Here's the drawing with two shaded views (mm, measured from the low corner). I have some questions. A direction names the side the tool comes from. Give positions to 0.01 mm unless a question says otherwise; leave off trailing zeros. Write each loop counter-clockwise with the first axis right and the second up, starting at its lowest first coordinate (ties: lowest second). Pieces come first, ordered by that corner, then holes. Notation, with made-up numbers: M 37.5,64 L 58.5,64 A5 cw 58.5,72 Z; hole C -14.5,48.25 d2. An arc over 180 degrees is marked long. Use one line per item in the form item = value.
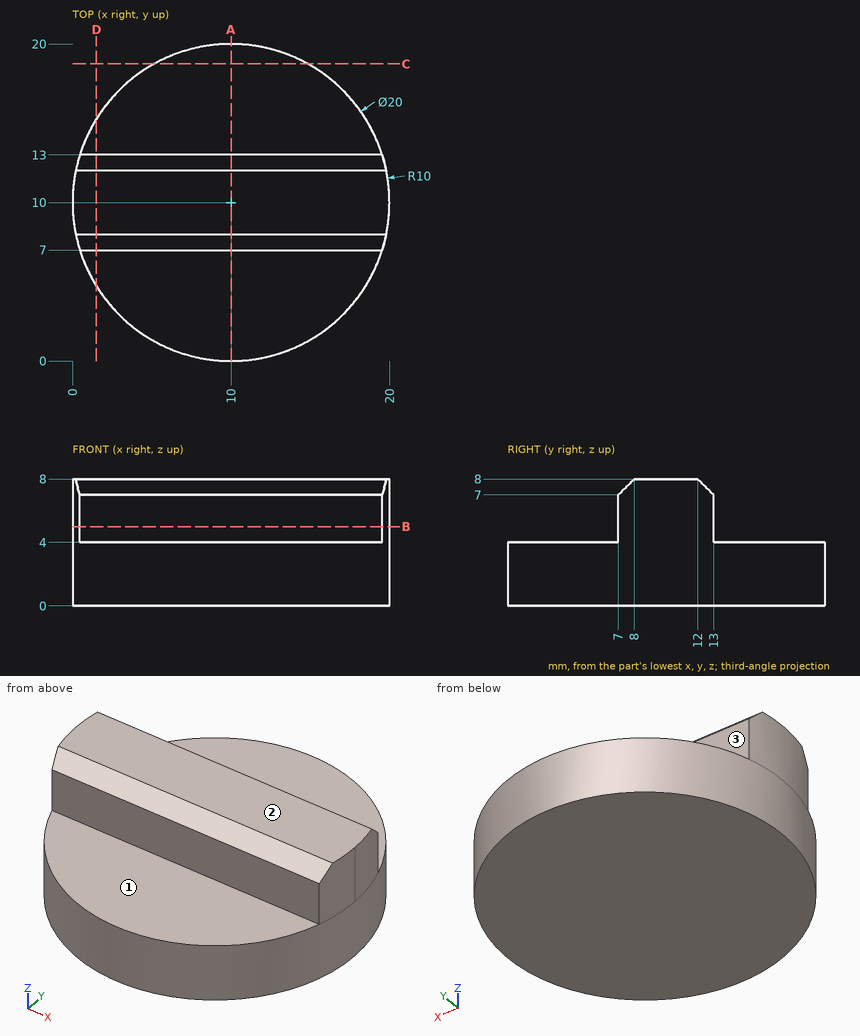
1) For pin 1 Ø2.5 at (x, z) = (10.5, 5) entering from +Y; pin 2 Ø1.5 at (x, z) = (6, 5.5) entering from -Y; pin 3 Ø1.5 at (x, z) = (5.5, 3) entering from +Y; pin 4 Ø3.5 at (x, y) = (6, 3.5) entering from +Z, each with a flat end and sliding along its axis, tell me the tip position at first contact or that it passes through.
Checked values:
pin_1 = 20
pin_2 = 7
pin_3 = 19.27
pin_4 = 4
2) If I drill on L1, parallel to Z at x = 8, y = 17; L2, parallel to Y at x = 2.5, z = 6.5; L3, parallel to X at y = 13, z = 0.5, over which ranges is the centre line in solid material (lowest first)?
Checked values:
L1 = 0 to 4
L2 = 7 to 13
L3 = 0.46 to 19.54
3) For the marked faces 1, 2 and 3, which set-ups out of +Z, -Z, +X, -X, +Y, -Y let a thin tool reach every point of the face, with its end or its side?
Checked values:
face_1 = +Z, +X, -X, -Y
face_2 = +Z, +X, -X, +Y, -Y
face_3 = +Z, +X, -X, +Y
4) I want a section at C-C, the plane y = 18.75. Please give me the cut outline in (x, z).
Checked values:
outline = M 5.16,0 L 14.84,0 L 14.84,4 L 5.16,4 Z
5) I want a section at B-B, the plane z = 5. Please give me the cut outline in (x, y), plus the area to 3 significant figures.
Checked values:
outline = M 0.46,7 L 19.54,7 A10 ccw 20,10 A10 ccw 19.54,13 L 0.46,13 A10 ccw Z
area = 118 mm2
6) I want a section at A-A, the plane x = 10. Please give me the cut outline in (y, z).
Checked values:
outline = M 0,0 L 20,0 L 20,4 L 13,4 L 13,7 L 12,8 L 8,8 L 7,7 L 7,4 L 0,4 Z
7) I want a section at D-D, the plane x = 1.5. Please give me the cut outline in (y, z).
Checked values:
outline = M 4.73,0 L 15.27,0 L 15.27,4 L 13,4 L 13,7 L 12,8 L 8,8 L 7,7 L 7,4 L 4.73,4 Z
